The model under review builds one solid part; all positions refer to its coordinate system, in mm. A direction names the side the tool comes from. Give positions to 0.01 mm unless a question says otherwise; leave off trailing zeros. Order: outer loops, then holes, each group sorted by start corner. A loop starts at its lowest first (then second) coordinate and runs counter-clockwise, first axis right, second up. Notation, with made-up numbers: (66, 1) -> (108, 1) arc R10 cw to (108, 11) -> close; hole circle Ø1 at (44, -20). An arc over 180 degrees is marked (long way). Answer as a JSON object with one key per item and string values. Group by question number.
from build123d import *

# Parameters (mm, degrees)
CROQUIS1_R              = 11.5
CROQUIS1_R_2            = 4.35
CROQUIS1_R_3            = 1.7000000000000004
SALIENTE_EXTRUIR1_DEPTH = 3.5
CROQUIS2_R              = 5.35
CROQUIS2_R_2            = 4.35
SALIENTE_EXTRUIR2_DEPTH = 13
CORTAR_EXTRUIR1_START   = -5
CORTAR_EXTRUIR1_DEPTH   = 5
CROQUIS4_R              = 5.275
CROQUIS4_R_2            = 4.35
CORTAR_EXTRUIR2_DEPTH   = 2
REDONDEO1_R             = 0.6
REDONDEO2_R             = 0.5
SALIENTE_EXTRUIR3_DEPTH = 3.5


with BuildPart() as part:
    # Croquis1 → Saliente-Extruir1 (new body)
    with BuildSketch(Plane(origin=(0, 0, 0), x_dir=(1, 0, 0), z_dir=(0, 1, 0))):
        with Locations(Location((1.731948e-11, 0, 0), (0, 0, 270))):
            Circle(CROQUIS1_R)
        with Locations(Location((1.731948e-11, 0, 0), (0, 0, 270))):
            Circle(CROQUIS1_R_2, mode=Mode.SUBTRACT)
        with Locations(Location((5.656854249492441, 5.65685424949238, 0), (0, 0, 270))):
            Circle(CROQUIS1_R_3, mode=Mode.SUBTRACT)
        with Locations(Location((-5.656854249492318, 5.656854249492381, 0), (0, 0, 270))):
            Circle(CROQUIS1_R_3, mode=Mode.SUBTRACT)
        with Locations(Location((-5.656854249492318, -5.656854249492381, 0), (0, 0, 270))):
            Circle(CROQUIS1_R_3, mode=Mode.SUBTRACT)
        with Locations(Location((5.656854249492441, -5.65685424949238, 0), (0, 0, 270))):
            Circle(CROQUIS1_R_3, mode=Mode.SUBTRACT)
    extrude(amount=SALIENTE_EXTRUIR1_DEPTH)

    # Croquis2 → Saliente-Extruir2 (add)
    with BuildSketch(Plane(origin=(0, 3.5, 0), x_dir=(1, 0, 0), z_dir=(0, 1, 0))):
        with Locations(Location((1.731948e-11, 0, 0), (0, 0, 90))):
            Circle(CROQUIS2_R)
        with Locations(Location((1.731948e-11, 0, 0), (0, 0, 270))):
            Circle(CROQUIS2_R_2, mode=Mode.SUBTRACT)
    extrude(amount=SALIENTE_EXTRUIR2_DEPTH)

    # Croquis3 → Cortar-Extruir1 (cut)
    with BuildSketch(Plane(origin=(0, 16.5, 0), x_dir=(1, 0, 0), z_dir=(0, 1, 0)).offset(CORTAR_EXTRUIR1_START)):
        with BuildLine():
            Line((1.732086e-11, 5.35), (1.732072e-11, 4.35))
            ThreePointArc((1.732072e-11, 4.35), (3.0759144981543076, 3.0759144981369877), (4.34999999998268, 0))
            Line((4.34999999998268, 0), (5.34999999998268, 0))
            ThreePointArc((5.34999999998268, 0), (3.783021279340855, 3.783021279323535), (1.732086e-11, 5.35))
        make_face()
        with BuildLine():
            Line((1.732086e-11, -5.35), (1.732072e-11, -4.35))
            ThreePointArc((1.732072e-11, -4.35), (-3.075914498144163, -3.075914498161481), (-4.34999999998268, 0))
            Line((-4.34999999998268, 0), (-5.34999999998268, 0))
            ThreePointArc((-5.34999999998268, 0), (-3.7830212793307103, -3.7830212793480285), (1.732086e-11, -5.35))
        make_face()
    extrude(amount=CORTAR_EXTRUIR1_DEPTH, mode=Mode.SUBTRACT)

    # Croquis4 → Cortar-Extruir2 (cut)
    with BuildSketch(Plane.XZ):
        with Locations(Location((1.731948e-11, 0, 0), (0, 0, 270))):
            Circle(CROQUIS4_R)
        with Locations(Location((1.731948e-11, 0, 0), (0, 0, 270))):
            Circle(CROQUIS4_R_2, mode=Mode.SUBTRACT)
    extrude(amount=-CORTAR_EXTRUIR2_DEPTH, mode=Mode.SUBTRACT)

    # Redondeo1
    redondeo1_edges = [part.edges().sort_by_distance(p)[0] for p in [
        (1.732109e-11, 0, 5.275),
    ]]
    fillet(redondeo1_edges, radius=REDONDEO1_R)

    # Redondeo2
    # the kernel refuses this fillet: 0.5 mm, written as the material it takes off along each edge
    with BuildSketch(Plane(origin=(-4.34999999998268, 11.5, -2.1e-16), x_dir=(0.05161519234821224, 0, -0.9986670475783493), z_dir=(0, 1, 0))) as redondeo2_piece_1:
        with BuildLine():
            CenterArc((0.4748597696035476, 0.49933352378917434), REDONDEO2_R, 182.9586473758917, 84.08270524821648)
            Line((-0.02447375418562714, 0.4735259276150691), (0, 0))
            ThreePointArc((0, 0), (0.22452608671472166, 0.00579834303418057), (0.44905217342944187, 0))
        make_face()
    extrude(amount=6.185394894032285, mode=Mode.SUBTRACT)
    with BuildSketch(Plane(origin=(-5.34999999998268, 11.5, 0), x_dir=(1, 0, 0), z_dir=(0, 1, 0))) as redondeo2_piece_2:
        with BuildLine():
            CenterArc((0.5258420423870858, 0.5), REDONDEO2_R, 174.0827052482164, 95.91729475178363)
            ThreePointArc((0.02850617046822901, 0.5515463917525775), (0.00713129545583069, 0.2761412790629337), (0, 0))
            Line((0, 0), (0.5258420423870858, 0))
        make_face()
    extrude(amount=6.380706395314668, mode=Mode.SUBTRACT)
    with BuildSketch(Plane(origin=(1.7321e-11, 11.5, 5.35), x_dir=(-3.5e-16, 0, -1), z_dir=(0, 1, 0))) as redondeo2_piece_3:
        with BuildLine():
            CenterArc((0.5258420423870855, -0.5), REDONDEO2_R, 89.99999999999997, 95.91729475178352)
            ThreePointArc((0.02850617046822881, -0.5515463917525766), (0.00713129545583059, -0.27614127906293173), (0, 0))
            Line((0, 0), (0.5258420423870858, 0))
        make_face()
    extrude(amount=6.3807063953146645, mode=Mode.SUBTRACT)
    with BuildSketch(Plane(origin=(1.731868e-11, 11.5, 4.35), x_dir=(0.9986670475783493, 0, -0.051615192348211894), z_dir=(0, 1, 0))) as redondeo2_piece_4:
        with BuildLine():
            CenterArc((0.474859769603551, -0.49933352378917434), REDONDEO2_R, 92.95864737589183, 84.08270524821639)
            Line((-0.0244737541856237, -0.4735259276150684), (0, 0))
            ThreePointArc((0, 0), (0.2245260867147224, -0.00579834303418053), (0.4490521734294448, 0))
        make_face()
    extrude(amount=6.185394894032285, mode=Mode.SUBTRACT)
    with BuildSketch(Plane(origin=(1.732072e-11, 11.5, -4.35), x_dir=(-0.9986670475783493, 0, 0.05161519234821218), z_dir=(0, 1, 0))) as redondeo2_piece_5:
        with BuildLine():
            CenterArc((0.474859769603548, -0.49933352378917434), REDONDEO2_R, 92.95864737589177, 84.08270524821641)
            Line((-0.02447375418562666, -0.47352592761506823), (0, 0))
            ThreePointArc((0, 0), (0.22452608671472019, -0.00579834303418048), (0.4490521734294423, 0))
        make_face()
    extrude(amount=6.185394894032285, mode=Mode.SUBTRACT)
    with BuildSketch(Plane(origin=(1.731981e-11, 11.5, -5.35), x_dir=(1.91e-15, 0, 1), z_dir=(0, 1, 0))) as redondeo2_piece_6:
        with BuildLine():
            CenterArc((0.5258420423870848, -0.5), REDONDEO2_R, 89.99999999999989, 95.91729475178357)
            ThreePointArc((0.02850617046822795, -0.5515463917525762), (0.00713129545583016, -0.2761412790629328), (0, 0))
            Line((0, 0), (0.5258420423870858, 0))
        make_face()
    extrude(amount=6.3807063953146645, mode=Mode.SUBTRACT)
    with BuildSketch(Plane(origin=(4.34999999998268, 11.5, 1.9e-16), x_dir=(-0.05161519227127975, 0, 0.9986670475823255), z_dir=(0, 1, 0))) as redondeo2_piece_7:
        with BuildLine():
            CenterArc((0.47485976964022647, 0.4993335237871862), REDONDEO2_R, 182.95864737147792, 84.08270524821648)
            Line((-0.02447375415093636, 0.4735259276515472), (0, 0))
            ThreePointArc((0, 0), (0.22452608671427532, 0.00579834305147695), (0.44905217342765447, 0))
        make_face()
    extrude(amount=6.1853948941188825, mode=Mode.SUBTRACT)
    with BuildSketch(Plane(origin=(5.34999999998268, 11.5, 0), x_dir=(-1, 0, 0), z_dir=(0, 1, 0))) as redondeo2_piece_8:
        with BuildLine():
            CenterArc((0.5258420423524468, 0.5), REDONDEO2_R, 174.08270524821663, 95.9172947517834)
            ThreePointArc((0.02850617043358916, 0.5515463917525757), (0.00713129542123792, 0.2761412790638253), (0, 0))
            Line((0, 0), (0.5258420423524468, 0))
        make_face()
    extrude(amount=6.380706395310192, mode=Mode.SUBTRACT)

    # Croquis5 → Saliente-Extruir3 (add)
    with BuildSketch(Plane(origin=(0, 3.5, 0), x_dir=(1, 0, 0), z_dir=(0, 1, 0))):
        with BuildLine():
            Line((-4.867801495370659, 2.219686599837588), (-10.46349854147086, 4.7712889529219185))
            ThreePointArc((-10.46349854147086, 4.7712889529219185), (-11.49999999998268, 1.41e-15), (-10.46349854147086, -4.771288952921916))
            Line((-10.46349854147086, -4.771288952921914), (-4.86780149537066, -2.219686599837586))
            ThreePointArc((-4.86780149537066, -2.219686599837586), (-5.34999999998268, 8.9e-16), (-4.86780149537066, 2.219686599837588))
        make_face()
        with BuildLine():
            Line((-2.2196865998351183, -4.867801495381207), (-4.77128895293652, -10.463498541473625))
            ThreePointArc((-4.771288952936522, -10.463498541473623), (-6.77758e-12, -11.5), (4.771288952927311, -10.463498541493617))
            Line((4.771288952927309, -10.46349854149362), (2.2196865998493576, -4.86780149539051))
            ThreePointArc((2.219686599849358, -4.867801495390509), (6.10956e-12, -5.35), (-2.219686599835118, -4.867801495381206))
        make_face()
        with BuildLine():
            ThreePointArc((11.50000000001732, 0), (11.237887551221265, 2.4412872396535783), (10.463498541496383, 4.771288952941911))
            Line((10.463498541496381, 4.7712889529419105), (4.867801495401058, 2.2196865998468893))
            ThreePointArc((4.867801495401059, 2.2196865998468898), (5.228060730360026, 1.1357292810562294), (5.350000000017321, -1.1e-16))
            ThreePointArc((5.350000000017321, -1.1e-16), (5.228060730360026, -1.1357292810562303), (4.867801495401057, -2.2196865998468898))
            Line((4.867801495401058, -2.2196865998468898), (10.463498541496381, -4.771288952941912))
            ThreePointArc((10.463498541496378, -4.7712889529419185), (11.237887551221265, -2.4412872396535787), (11.50000000001732, -2.82e-15))
        make_face()
        with BuildLine():
            ThreePointArc((4.771288952927309, 10.46349854149362), (-6.77732e-12, 11.5), (-4.771288952936519, 10.463498541473625))
            Line((-4.771288952936519, 10.463498541473623), (-2.2196865998351187, 4.867801495381207))
            ThreePointArc((-2.219686599835118, 4.867801495381207), (6.10867e-12, 5.35), (2.219686599849357, 4.86780149539051))
            Line((2.2196865998493576, 4.86780149539051), (4.771288952927309, 10.46349854149362))
        make_face()
    extrude(amount=SALIENTE_EXTRUIR3_DEPTH)


solid = part.part
1. Take a section at A-A on y = 10.75. Give the boundary of the cut face in (x, z), plus the area to 3 significant figures.
2. Take a section at C-C on z = 9. Give the boundary of the cut face in (x, y).
3. For pin 1 (3.5 mm diameter, centred on x = -2, z = 8, fed in from +Y); pin 2 (2.5 mm diameter, centred on x = 5.66, z = -5.66, fed in from -Y); pin 3 (2.5 mm diameter, centred on x = 6, z = -8, fed in from +Y); pin 4 (1.5 mm diameter, centred on x = -6.5, y = 4, fed in from -Z), all flat-tipped, find the tip position at first contact; note any pin that passes through.
4. Take a section at B-B on x = 7. Give the boundary of the cut face in (y, z).
5. Draft analysis for pull direction Z (two halves, no side actions). For faces 6 (the flat face through (3.51, 5.23, 7.7)), 7 (the flat face through (7.7, 5.23, -3.51)), 8 (the flat face through (0, 7, -8)), 9 (the flat face through (-7.7, 5.23, 3.51)), state which applies: pulls with the +Z half, pulls with the -Z half, needs draft (parallel to the pull), parting line crosses it, or undercut.
6. For probe 1 along X at (y, z) = (1.15, 0) (3 decimals); probe 2 along Y at (x, z) = (5.25, 9.25); probe 3 along Y at (x, z) = (-7, -1), list the stretches that pass through material, from the lowest coordinate up. Write a range as [from, to].
7. Machinability: for faces 1 (the flat face through (7.63, 5.23, 3.48)), 2 (the flat face through (-7, 3.5, -7)), 3 (the flat face through (3.2, 2, 3.2)), 4 (the flat face through (-3.48, 5.23, 7.63)), 5 (the cylindrical face through (-6.308, 1.726, 7.227)), which of the approach directions +Z, -Z, +X, -X, +Y, -Y give a long, thin tool a straight path to every point of the face, cutting with its end or side? Answer none if there is none.
Checks:
{
 "1": {"outline": "circle Ø10.7 at (0, 0); hole circle Ø8.7 at (0, 0)", "area": "30.5 mm2"},
 "2": {"outline": "(-7.16, 0) -> (7.16, 0) -> (7.16, 3.5) -> (4.1, 3.5) -> (4.1, 7) -> (-4.1, 7) -> (-4.1, 3.5) -> (-7.16, 3.5) -> close"},
 "3": {"pin 1": "stops at y = 7", "pin 2": "passes through", "pin 3": "stops at y = 3.5", "pin 4": "stops at z = -9.85"},
 "4": {"outline": "(0, -9.12) -> (3.5, -9.12) -> (3.5, -6.7) -> (0, -6.7) -> close; (0, -4.61) -> (3.5, -4.61) -> (3.5, -3.19) -> (7, -3.19) -> (7, 3.19) -> (3.5, 3.19) -> (3.5, 4.61) -> (0, 4.61) -> close; (0, 6.7) -> (3.5, 6.7) -> (3.5, 9.12) -> (0, 9.12) -> close"},
 "5": {"face 6": "undercut", "face 7": "pulls with the -Z half", "face 8": "needs draft", "face 9": "pulls with the +Z half"},
 "6": {"probe 1": "x = [-11.5, -5.275], [5.275, 11.5]", "probe 2": "y = [0, 3.5]", "probe 3": "y = [0, 7]"},
 "7": {"face 1": "+Z, +Y", "face 2": "+Y", "face 3": "-Y", "face 4": "-X, +Y", "face 5": "+Y, -Y"}
}
